CAD build for the part. Positions are in the model's coordinates, mm. A direction names the side the tool comes from. Coordinates: 2 decimals unless noted, no trailing zeros. Order: outer loops, then holes, each group sorted by start corner. A loop starts at its lowest first (then second) coordinate and runs counter-clockwise, first axis right, second up. Notation, with made-up numbers: M 59,23 L 86,23 A24 cw 86,44 Z; hole C 66,-11 d9. An arc over 180 degrees is marked long. Write item = value, one per line.
from build123d import *

# Parameters (mm, degrees)
SKETCH1_W              = 260
SKETCH1_H              = 49
BOSS_EXTRUDE1_DEPTH    = 6
SKETCH2_W              = 120
SKETCH2_H              = 6
CUT_EXTRUDE1_DEPTH     = 6
M8X1_25_TAPPED_HOLE1_D = 6.8
CUT_EXTRUDE2_REACH     = 141.058
SKETCH5_W              = 6
SKETCH5_H              = 23
SKETCH6_W              = 120
SKETCH6_H              = 6
BOSS_EXTRUDE2_DEPTH    = 6


with BuildPart() as part:
    # Sketch1 → Boss-Extrude1 (new body)
    with BuildSketch(Plane.XY):
        with Locations((0, 24.5)):
            Rectangle(SKETCH1_W, SKETCH1_H)
    extrude(amount=BOSS_EXTRUDE1_DEPTH)

    # Sketch2 → Cut-Extrude1 (cut)
    with BuildSketch(Plane(origin=(0, 0, 0), x_dir=(-1, 0, 0), z_dir=(0, 0, -1))):
        with Locations((-70, 46)):
            Rectangle(SKETCH2_W, SKETCH2_H)
        with Locations((70, 46)):
            Rectangle(SKETCH2_W, SKETCH2_H)
    extrude(amount=-CUT_EXTRUDE1_DEPTH, mode=Mode.SUBTRACT)

    # M8x1.25 Tapped Hole1 (through all)
    with Locations(Plane(origin=(0, 0, 0), x_dir=(-1, 0, 0), z_dir=(0, 0, -1))):
        with Locations((0, 39)):
            Hole(M8X1_25_TAPPED_HOLE1_D / 2)

    # Sketch5 → Cut-Extrude2 (cut, up to next)
    with BuildSketch(Plane(origin=(0, 0, 0), x_dir=(-1, 0, 0), z_dir=(0, 0, -1)), mode=Mode.PRIVATE) as cut_extrude2_sk1:
        with Locations((-127, 31.5)):
            Rectangle(SKETCH5_W, SKETCH5_H)
    cut_extrude2_tool1 = extrude(cut_extrude2_sk1.sketch, amount=-CUT_EXTRUDE2_REACH, mode=Mode.PRIVATE) & part.part
    # Sketch5 → Cut-Extrude2 (cut, up to next)
    with BuildSketch(Plane(origin=(0, 0, 0), x_dir=(-1, 0, 0), z_dir=(0, 0, -1)), mode=Mode.PRIVATE) as cut_extrude2_sk2:
        with Locations((127, 31.5)):
            Rectangle(SKETCH5_W, SKETCH5_H)
    cut_extrude2_tool2 = extrude(cut_extrude2_sk2.sketch, amount=-CUT_EXTRUDE2_REACH, mode=Mode.PRIVATE) & part.part
    add(cut_extrude2_tool1.solids().sort_by_distance((127, 31.5, 0))[0], mode=Mode.SUBTRACT)
    add(cut_extrude2_tool2.solids().sort_by_distance((-127, 31.5, 0))[0], mode=Mode.SUBTRACT)

    # Sketch6 → Boss-Extrude2 (add)
    with BuildSketch(Plane(origin=(0, 0, 0), x_dir=(-1, 0, 0), z_dir=(0, 0, -1))):
        with Locations((0, -3)):
            Rectangle(SKETCH6_W, SKETCH6_H)
    extrude(amount=-BOSS_EXTRUDE2_DEPTH)


solid = part.part
(1) Slice it at A-A, the plane x = 0. Write the cut outline in (y, z).
Evaluation:
outline = M -6,0 L 35.6,0 L 35.6,6 L -6,6 Z; M 42.4,0 L 49,0 L 49,6 L 42.4,6 Z
(2) Pull direction X, two halves, no side cores. Call faces 1 (the face through (-60, -3, 3)), 2 (the face through (10, 46, 3)), 3 (the face through (-0.44, 42.37, 3.04)), 4 (the face through (68, 43, 3)): +X half, -X half, draft (parallel to the pull), parting line (faces both ways), or undercut.
Evaluation:
face_1 = -X half
face_2 = +X half
face_3 = undercut
face_4 = draft
(3) Slice it at D-D, the plane x = -57. Write the cut outline in (y, z).
Evaluation:
outline = M -6,0 L 43,0 L 43,6 L -6,6 Z
(4) Tool access for faces 5 (the face through (95, 0, 3)), 6 (the face through (127, 20, 3)), 7 (the face through (-95, 0, 3)), 8 (the face through (-66, 43, 3)): list every direction of +Z, -Z, +X, -X, +Y, -Y with a clear straight run to the whole face (end or side of a thin tool).
Evaluation:
face_5 = +Z, -Z, +X, -Y
face_6 = +Z, -Z, +X, +Y
face_7 = +Z, -Z, -X, -Y
face_8 = +Z, -Z, -X, +Y
(5) Slice it at C-C, the plane z = 1.75. Write the cut outline in (x, y).
Evaluation:
outline = M -130,0 L -60,0 L -60,-6 L 60,-6 L 60,0 L 130,0 L 130,20 L 124,20 L 124,43 L 10,43 L 10,49 L -10,49 L -10,43 L -124,43 L -124,20 L -130,20 Z; hole C 0,39 d6.8
(6) Wall check: line 1 (Y direction, x = 0, z = 2.9); line 2 (Y direction, x = 83, z = 1.2); line 3 (Y direction, x = -11, z = 1.9). Give the ranges that are in metal, low to high. Write a range as from..to.
Evaluation:
line_1 = -6..35.6, 42.4..49
line_2 = 0..43
line_3 = -6..43
(7) Slice it at B-B, the plane y = 39. Write the cut outline in (x, z).
Evaluation:
outline = M -124,0 L -3.4,0 L -3.4,6 L -124,6 Z; M 3.4,0 L 124,0 L 124,6 L 3.4,6 Z
(8) Pin check, flat tips, straight feed: pin 1 Ø3 at (x, z) = (128.5, 1.5) entering from +Y; pin 2 Ø3 at (y, z) = (45, 3.5) entering from +X; pin 3 Ø2 at (x, z) = (84, 1.5) entering from -Y. Stop position of each tip, or through.
Evaluation:
pin_1 = 20
pin_2 = 10
pin_3 = 0
